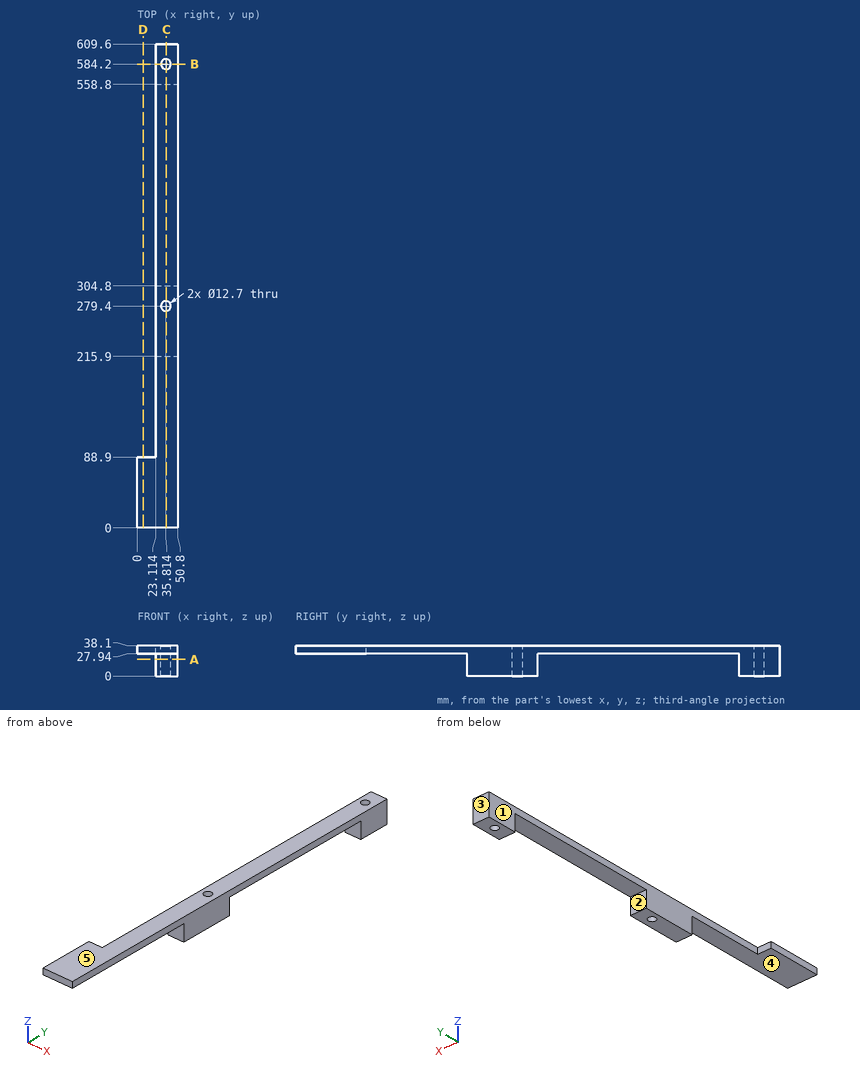
The drawing under review shows one solid part. Ordinate dimensions are in mm from its lowest x, y, z. A direction names the side the tool comes from. Give positions to 0.01 mm unless a question says otherwise; leave off trailing zeros. Order: outer loops, then holes, each group sorted by start corner. A loop starts at its lowest first (then second) coordinate and runs counter-clockwise, first axis right, second up. Notation, with made-up numbers: M -5,28.5 L 37,28.5 A15 ccw 37,48.5 Z; hole C 13.25,82 d7. An arc over 180 degrees is marked long. One line per question, with ' | ' between items. Start each with the question number.
Q1. For pin 1 Ø8 at (y, z) = (369, 25.5) entering from -X; pin 2 Ø14 at (x, y) = (36.5, 459.5) entering from -Z; pin 3 Ø10 at (x, y) = (35.814, 584.2) entering from -Z; pin 4 Ø8.5 at (x, z) = (30.5, 16.5) entering from -Y, all flat-tipped, find the tip position at first contact; note any pin that passes through.
Q2. Machinability: for the marked faces 4 and 5, which of the approach directions +Z, -Z, +X, -X, +Y, -Y give a long, thin tool a straight path to every point of the face, cutting with its end or side? Answer none if there is none.
Q3. We need section A-A (z = 21). Write out the cut boundary in (x, y), plus the area to 3 significant figures.
Q4. We need section C-C (x = 36.5). Write out the cut boundary in (y, z).
Q5. For L1, parallel to Y at x = 27, z = 3; L2, parallel to Y at x = 35, z = 13.5; L3, parallel to X at y = 584.2, z = 20, list the stretches that pass through material, from the lowest coordinate up. Write a range as [from, to].
Q6. We need section D-D (x = 7). Write out the cut boundary in (y, z).
Q7. The part is to be moulded in two halves that separate along Y. For the marked faces 1, 2 and 3, say which applies: +Y half, -Y half, draft (parallel to the pull), parting line (faces both ways), or undercut.
Q8. We need section B-B (y = 584.2). Write out the cut boundary in (x, z), plus the area to 3 significant figures.
Returned:
1) pin 1: x = 23.11 | pin 2: z = 27.94 | pin 3: through | pin 4: y = 215.9
2) face 4: -Z, +X, -X, -Y | face 5: +Z, +X, -X, +Y, -Y
3) outline: M 23.11,215.9 L 50.8,215.9 L 50.8,304.8 L 23.11,304.8 Z; M 23.11,558.8 L 50.8,558.8 L 50.8,609.6 L 23.11,609.6 Z; hole C 35.81,279.4 d12.7; hole C 35.81,584.2 d12.7 | area: 3,610 mm2
4) outline: M 0,27.94 L 215.9,27.94 L 215.9,0 L 273.09,0 L 273.09,38.1 L 0,38.1 Z; M 285.71,0 L 304.8,0 L 304.8,27.94 L 558.8,27.94 L 558.8,0 L 577.89,0 L 577.89,38.1 L 285.71,38.1 Z; M 590.51,0 L 609.6,0 L 609.6,38.1 L 590.51,38.1 Z
5) L1: [215.9, 304.8], [558.8, 609.6] | L2: [215.9, 273.1], [285.7, 304.8], [558.8, 577.9], [590.5, 609.6] | L3: [23.11, 29.46], [42.16, 50.8]
6) outline: M 0,27.94 L 88.9,27.94 L 88.9,38.1 L 0,38.1 Z
7) face 1: draft | face 2: undercut | face 3: +Y half
8) outline: M 23.11,0 L 29.46,0 L 29.46,38.1 L 23.11,38.1 Z; M 42.16,0 L 50.8,0 L 50.8,38.1 L 42.16,38.1 Z | area: 571 mm2
